Autodesk Inventor part; units mm, degrees
ref_plane "YZ Plane" through (0, 0, 0) normal (1, 0, 0) x (0, 1, 0)
ref_plane "XZ Plane" through (0, 0, 0) normal (0, 1, 0) x (-1, 0, 0)
ref_plane "XY Plane" through (0, 0, 0) normal (0, 0, 1) x (1, 0, 0)
sketch "Sketch1" plane through (0, 0, 0) normal (0, 1, 0) x (-1, 0, 0)
  line L0 (0, 0) -> (20, 0)
  line L1 (20, 0) -> (20, -20)
  line L2 (20, -20) -> (0, -20)
  line L3 (0, -20) -> (0, 0)
  line L4 (20, 0) -> (18, 0)
  line L5 (18, 0) -> (18, -2)
  line L6 (18, -2) -> (20, -2)
  line L7 (20, -2) -> (20, 0)
  line L8 (20, -20) -> (18, -20)
  line L9 (18, -20) -> (18, -18)
  line L10 (18, -18) -> (20, -18)
  line L11 (20, -18) -> (20, -20)
  line L12 (0, 0) -> (2, 0)
  line L13 (2, 0) -> (2, -2)
  line L14 (2, -2) -> (0, -2)
  line L15 (0, -2) -> (0, 0)
  line L16 (0, -20) -> (2, -20)
  line L17 (2, -20) -> (2, -18)
  line L18 (2, -18) -> (0, -18)
  line L19 (0, -18) -> (0, -20)
  circle A0 centre (2, -2) radius 1
  circle A1 centre (2, -18) radius 1
  circle A2 centre (18, -18) radius 1
  circle A3 centre (18, -2) radius 1
  line L20 (0, 0) -> (-10, 0)
  line L21 (-10, 0) -> (-10, -20)
  line L22 (-10, -20) -> (0, -20)
  line L23 (0, -20) -> (0, 0)
  dimension "d0" = 20
  dimension "d1" = 20
  dimension "d2" = 2
  dimension "d3" = 2
  dimension "d4" = 2
  dimension "d5" = 2
  dimension "d6" = 2
  dimension "d7" = 2
  dimension "d8" = 2
  dimension "d9" = 2
  dimension "d10" = 2
  dimension "d11" = 2
  dimension "d12" = 2
  dimension "d13" = 2
  dimension "d16" = 10
extrude "Extrusion1" add sketch "Sketch1" along normal blind 3 contours L0 L13 A0 L14 L3 | L3 L22 L21 L20 | L0 L5 A3 L6 L1 L10 A2 L9 L2 L17 A1 L18 L3 L14 A0 L13 | L0 L1 L6 A3 L5 | L18 A1 L17 L2 L3 | L1 L2 L9 A2 L10
sketch "Sketch2" plane through (0, 0, 0) normal (0, -1, 0) x (1, 0, 0)
  line L0 (-20, 0) -> (10, 0)
  line L1 (10, 0) -> (-0.35, 0)
  line L2 (-0.35, 0) -> (-0.35, -8.5)
  line L3 (-0.35, -8.5) -> (10, -8.5)
  line L4 (10, -8.5) -> (10, 0)
  circle A0 centre (-0.35, -8.5) radius 3.05
  circle A1 centre (-0.35, -8.5) radius 3.75
  point P0 (0, 0)
  dimension "d17" = 10.35
  dimension "d18" = 8.5
  dimension "d19" = 6.1
  dimension "d20" = 7.5
extrude "Extrusion2" add sketch "Sketch2" against normal blind 6 contours A1 L3 A0 L2 | L2 A0 L3 A1
sketch "Sketch3" plane through (-0.35, 6, -8.5) normal (0, 1, 0) x (-1, 0, 0)
  circle A0 centre (0, 0) radius 3.05
  circle A1 centre (0, 0) radius 3.05
  circle A2 centre (0, 0) radius 2.85
  point P0 (-0.35, 8.5)
  dimension "d23" = 5.7
extrude "Extrusion3" add sketch "Sketch3" against normal blind 0.3
sketch "Sketch4" plane through (-0.35, 6, -8.5) normal (0, 1, 0) x (-1, 0, 0)
  line L0 (-0.75, -4.5946) -> (0.75, -4.5946)
  line L1 (0.75, -4.5946) -> (0.75, 4.5946)
  line L2 (0.75, 4.5946) -> (-0.75, 4.5946)
  line L3 (-0.75, 4.5946) -> (-0.75, -4.5946)
  circle A0 centre (0, 0) radius 2.85
  line L4 (-0.75, -4.5946) -> (0.75, 4.5946) construction
  line L5 (0.75, -4.5946) -> (-0.75, 4.5946) construction
  point P0 (-0.35, 8.5)
  dimension "d26" = 1.5
extrude "Extrusion4" cut sketch "Sketch4" against normal blind 3 contours L3 A0 L1 L0 | L3 A0 L1 | L3 L2 L1 A0
properties part number "bearing_support"
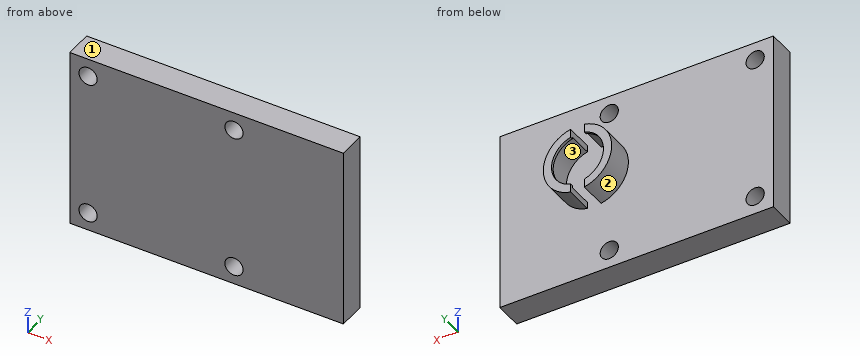
Geometry check sheet. Reference: the model listing, model coordinates, mm. Face numbers are marked on the shaded views. Round coordinates to 2 decimals unless told otherwise and drop trailing zeros. Order: outer loops, then holes, each group sorted by start corner. A loop starts at its lowest first (then second) coordinate and runs counter-clockwise, first axis right, second up. Notation, with made-up numbers: M -10,42.25 L 37,42.25 A29 cw 37,80.25 Z; hole C 72,34 d3. An arc over 180 degrees is marked long. Answer in a Markdown table with one row per item. Add a question column.
Item 1: Draft check along Z on the marked faces 1, 2 and 3. Enter one of: released by +Z, released by -Z, zero draft, split by the parting line, or undercut.
Item 2: Material ranges on L1, parallel to Z at x = -2, y = 1.2; L2, parallel to X at y = 1.7, z = -18; L3, parallel to Z at x = -2.5, y = 2.35, recorded low to high. Write a range as [from, to].
Item 3: Sectioned sample at D-D, the plane y = 1.5. Enter the section's corners in (x, z).
Item 4: Sectioned sample at B-B, the plane z = -18. Enter the section's corners in (x, y).
Item 5: Sectioned sample at A-A, the plane x = -18. Enter the section's corners in (y, z), plus the area to 3 significant figures.
Item 6: Depth check by flat-ended pin: pin 1 Ø0.5 at (y, z) = (4.5, -5) entering from -X; pin 2 Ø4 at (x, z) = (-10.5, -17.5) entering from +Y; pin 3 Ø0.7 at (y, z) = (4.5, -11.5) entering from -X; pin 4 Ø3 at (x, z) = (-2, -18) entering from -Y. Enter the tip coordinate at first touch or a pass-through.
Filled in:
| question | item | result |
|---|---|---|
| 1 | face 1 | released by +Z |
| 1 | face 2 | split by the parting line |
| 1 | face 3 | undercut |
| 2 | L1 | z = [-20, -19], [-17, -3], [-1, 0] |
| 2 | L2 | x = [-20, -19], [-17, -3], [-1, 10] |
| 2 | L3 | z = [-20, -18.87], [-17.13, -2.87], [-1.13, 0] |
| 3 | outline | M -20,-20 L 10,-20 L 10,0 L -20,0 Z; hole C -18,-18 d2; hole C -18,-2 d2; hole C -2,-18 d2; hole C -2,-2 d2 |
| 4 | outline | M -20,0 L -19,0 L -19,3 L -20,3 Z; M -17,0 L -3,0 L -3,3 L -17,3 Z; M -1,0 L 10,0 L 10,3 L -1,3 Z |
| 5 | outline | M 0,-20 L 3,-20 L 3,-19 L 0,-19 Z; M 0,-17 L 3,-17 L 3,-3 L 0,-3 Z; M 0,-1 L 3,-1 L 3,0 L 0,0 Z |
| 5 | area | 48.0 mm² |
| 6 | pin 1 | stops at x = -2.22 |
| 6 | pin 2 | stops at y = 3 |
| 6 | pin 3 | stops at x = -3 |
| 6 | pin 4 | stops at y = 0 |
